Could you check a few things on this model? Use its own coordinates, in mm. Face numbers are marked on the shaded views. A direction names the side the tool comes from. Coordinates: 2 decimals unless noted, no trailing zeros. Loops run counter-clockwise (first coordinate to the right, second up) from the corner with the lowest first, then second, coordinate; pieces in that order, holes last. Notation, with made-up numbers: (62.25, -10.75) - (75.25, -10.75) arc R16 ccw to (75.25, 1.25) - close; hole circle Ø10 at (88, 45). An arc over 180 degrees is marked (long way). Put each result on its own line as item: value. Start each with the question number.
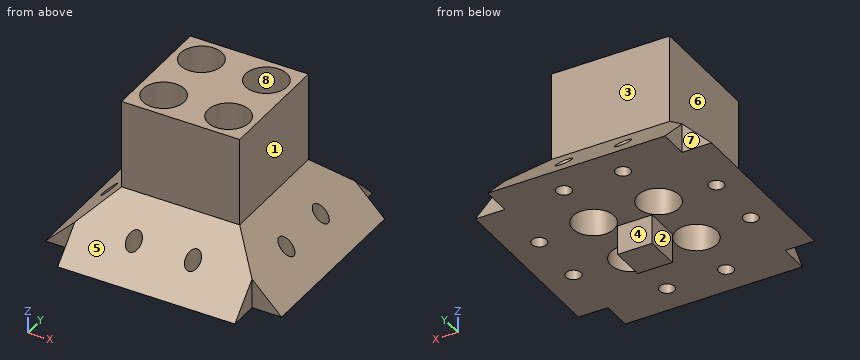
```python
from build123d import *

# Parameters (mm, degrees)
SKETCH_1_W                = 20
SKETCH_1_H                = 20
EXTRUDE_1_DEPTH           = 40
SKETCH_2_W                = 10
SKETCH_2_H                = 15
CUT_EXTRUDE_1_DEPTH       = 7.071067812
PATTERN_CIRCULAR_1_COUNT  = 4
SKETCH_5_R                = 3.5
CUT_EXTRUDE_2_DEPTH       = 25
CUT_EXTRUDE_3_DEPTH       = 5
SKETCH_9_W                = 5.878932188
SKETCH_9_H                = 5.878932188
CUT_EXTRUDE_5_DEPTH       = 5
SKETCH_11_W               = 10
SKETCH_11_H               = 30
EXTRUDE_2_DEPTH           = 10
CUT_EXTRUDE_6_DEPTH       = 30
SKETCH_13_R               = 1.25
CUT_EXTRUDE_7_DEPTH       = 10
PATTERN_CIRCULAR_2_COUNT  = 4
SKETCH_16_W               = 20
SKETCH_16_H               = 10
CUT_EXTRUDE_11_DEPTH      = 40
SKETCH_17_W               = 20
SKETCH_17_H               = 20
SKETCH_17_W_2             = 5.857864376
SKETCH_17_H_2             = 5.857864376
CUT_EXTRUDE_12_DEPTH      = 5
CUT_EXTRUDE_13_DEPTH      = 54.851648071
CUT_EXTRUDE_13_DEPTH_BACK = 10


with BuildPart() as part:
    # 스케치1 → 보스-돌출1 (new body)
    with BuildSketch(Plane.XY):
        Rectangle(SKETCH_1_W, SKETCH_1_H)
    extrude(amount=EXTRUDE_1_DEPTH)

    # 스케치2 → 컷-돌출1 (cut)
    with BuildSketch(Plane(origin=(10, 0, 0), x_dir=(0, 0, -1), z_dir=(1, 0, 0))):
        with Locations((-10, 0)):
            Rectangle(SKETCH_2_W, SKETCH_2_H)
    cut_extrude_1 = extrude(amount=-CUT_EXTRUDE_1_DEPTH, mode=Mode.SUBTRACT)

    # 원형 패턴1: 컷-돌출1 ×4 about axis
    pattern_circular_1_axis = Axis((0, 0, 0), (0, 0, 1))
    for i in range(1, PATTERN_CIRCULAR_1_COUNT):
        add(cut_extrude_1.rotate(pattern_circular_1_axis, i * 360 / PATTERN_CIRCULAR_1_COUNT), mode=Mode.SUBTRACT)

    # 스케치5 → 컷-돌출2 (cut)
    with BuildSketch(Plane.XY.offset(40)):
        with Locations((-5.5, 5.5)):
            Circle(SKETCH_5_R)
        with Locations((5.5, 5.5)):
            Circle(SKETCH_5_R)
        with Locations(Location((-5.5, -5.5, 0), (0, 0, 235.150095421))):
            Circle(SKETCH_5_R)
        with Locations(Location((5.5, -5.5, 0), (0, 0, 304.849904579))):
            Circle(SKETCH_5_R)
    extrude(amount=-CUT_EXTRUDE_2_DEPTH, mode=Mode.SUBTRACT)

    # 스케치6 → 컷-돌출3 (cut)
    with BuildSketch(Plane(origin=(0, 0, 0), x_dir=(-1, 0, 0), z_dir=(0, 0, -1))):
        Polygon((-14.808802863, -2.95), (-14.808802863, 2.95), (-2.95, 2.95), (-2.95, 12.360254216), (2.95, 12.360254216), (2.95, 2.95), (13.852115441, 2.95), (13.852115441, -2.95), (2.95, -2.95), (2.95, -13.975695818), (-2.95, -13.975695818), (-2.95, -2.95), align=None)
    extrude(amount=-CUT_EXTRUDE_3_DEPTH, mode=Mode.SUBTRACT)

    # 스케치9 → 컷-돌출5 (cut)
    with BuildSketch(Plane(origin=(0, 0, 5), x_dir=(-1, 0, 0), z_dir=(0, 0, -1))):
        with Locations((0.010533906, -0.010533906)):
            Rectangle(SKETCH_9_W, SKETCH_9_H)
    extrude(amount=-CUT_EXTRUDE_5_DEPTH, mode=Mode.SUBTRACT)

    # 스케치11 → 보스-돌출2 (add)
    with BuildSketch(Plane(origin=(10, 0, 0), x_dir=(0, 0, -1), z_dir=(1, 0, 0))):
        with Locations((-20, 0)):
            Rectangle(SKETCH_11_W, SKETCH_11_H)
    extrude_2 = extrude(amount=EXTRUDE_2_DEPTH)

    # 스케치12 → 컷-돌출6 (cut)
    with BuildSketch(Plane(origin=(0, 15, 0), x_dir=(1, 0, 0), z_dir=(0, 1, 0))):
        Polygon((20, -15), (10, -25), (20, -25), align=None)
    cut_extrude_6 = extrude(amount=-CUT_EXTRUDE_6_DEPTH, mode=Mode.SUBTRACT)

    # 스케치13 → 컷-돌출7 (cut)
    with BuildSketch(Plane(origin=(0, 0, 15), x_dir=(-1, 0, 0), z_dir=(0, 0, -1))):
        with Locations(Location((-15, -5, 0), (0, 0, 90))):
            Circle(SKETCH_13_R)
        with Locations(Location((-15, 5, 0), (0, 0, 90))):
            Circle(SKETCH_13_R)
    cut_extrude_7 = extrude(amount=-CUT_EXTRUDE_7_DEPTH, mode=Mode.SUBTRACT)

    # 원형 패턴2: 보스-돌출2, 컷-돌출6, 컷-돌출7 ×4 about axis
    pattern_circular_2_axis = Axis((0, 0, 0), (0, 0, 1))
    add([extrude_2.rotate(pattern_circular_2_axis, i * 360 / PATTERN_CIRCULAR_2_COUNT) for i in range(1, PATTERN_CIRCULAR_2_COUNT)])
    add([cut_extrude_6.rotate(pattern_circular_2_axis, i * 360 / PATTERN_CIRCULAR_2_COUNT) for i in range(1, PATTERN_CIRCULAR_2_COUNT)], mode=Mode.SUBTRACT)
    add([cut_extrude_7.rotate(pattern_circular_2_axis, i * 360 / PATTERN_CIRCULAR_2_COUNT) for i in range(1, PATTERN_CIRCULAR_2_COUNT)], mode=Mode.SUBTRACT)

    # 스케치16 → 컷-돌출11 (cut)
    with BuildSketch(Plane.XZ.offset(10)):
        with Locations((0, 5)):
            Rectangle(SKETCH_16_W, SKETCH_16_H)
    extrude(amount=-CUT_EXTRUDE_11_DEPTH, mode=Mode.SUBTRACT)

    # 스케치17 → 컷-돌출12 (cut)
    with BuildSketch(Plane(origin=(0, 0, 10), x_dir=(-1, 0, 0), z_dir=(0, 0, -1))):
        Rectangle(SKETCH_17_W, SKETCH_17_H)
        Rectangle(SKETCH_17_W_2, SKETCH_17_H_2, mode=Mode.SUBTRACT)
    extrude(amount=-CUT_EXTRUDE_12_DEPTH, mode=Mode.SUBTRACT)

    # 스케치18 → 컷-돌출13 (cut, two sides: drawn at the far end of the back side and taken through both)
    with BuildSketch(Plane.XZ.offset(-10).offset(-CUT_EXTRUDE_13_DEPTH_BACK)):
        Polygon((10, 25), (15, 25), (15, 20), align=None)
    extrude(amount=CUT_EXTRUDE_13_DEPTH + CUT_EXTRUDE_13_DEPTH_BACK, mode=Mode.SUBTRACT)


solid = part.part
```
(1) For pin 1 Ø3 at (x, y) = (5, 15) entering from -Z; pin 2 Ø5.5 at (y, z) = (16.5, 18.5) entering from -X; pin 3 Ø12 at (y, z) = (9, 35.5) entering from -X, each with a flat end and sliding along its axis, tell me the tip position at first contact or that it passes through.
(2) Which directions (+Z, -Z, +X, -X, +Y, -Y) give clear straight access to the entire face, cutting with the end or side of a thin tool? Please do the marked faces 1, 2, 3 and 4.
(3) I want a section at C-C on x = -5.5. List the corners of the cut face in (y, z) for me.
(4) I want a section at A-A on y = -5. List the corners of the cut face in (x, z) for me.
(5) I want a section at D-D on x = -0.5. List the corners of the cut face in (y, z) for me.
(6) I need wall thicknesses on L1, parallel to Y at x = -5, z = 19; L2, parallel to X at y = 8.5, z = 15.25; L3, parallel to Y at x = 8, z = 34.25. Which ranges of each line are inside material? Lowest first, please. Write a range as [from, to].
(7) If we mould it in two halves opening along Y, with no side actions, what happens to the marked faces 5, 6, 7 and 8? For each: pulls with the +Y half, pulls with the -Y half, needs draft (parallel to the pull), parting line crosses it, or undercut.
(8) I want a section at B-B on z = 37.75. List the corners of the cut face in (x, y) for me, and give its area (3 significant figures).
Answer sheet:
1. pin 1: stops at z = 15
1. pin 2: stops at x = -18.8
1. pin 3: stops at x = -10
2. face 1: +Z, +X, +Y, -Y
2. face 2: -Z, -X, +Y, -Y
2. face 3: +Z, +X, -X, +Y
2. face 4: -Z, +X, -X, +Y
3. outline: (-20, 15) - (-16.15, 15) - (-16.15, 18.85) - close; (-13.85, 15) - (-9, 15) - (-9, 40) - (-10, 40) - (-10, 25) - (-13.85, 21.15) - close; (-2, 15) - (2, 15) - (2, 40) - (-2, 40) - close; (9, 15) - (13.85, 15) - (13.85, 21.15) - (10, 25) - (10, 40) - (9, 40) - close; (16.15, 15) - (20, 15) - (16.15, 18.85) - close
4. outline: (-20, 15) - (-16.25, 15) - (-16.25, 18.75) - close; (-13.75, 15) - (-8.96, 15) - (-8.96, 40) - (-10, 40) - (-10, 25) - (-13.75, 21.25) - close; (-2.04, 15) - (2.04, 15) - (2.04, 40) - (-2.04, 40) - close; (8.96, 15) - (13.75, 15) - (13.75, 21.25) - (10, 25) - (10, 40) - (8.96, 40) - close; (16.25, 15) - (20, 15) - (16.25, 18.75) - close
5. outline: (-20, 15) - (-2.93, 15) - (-2.93, 10) - (2.93, 10) - (2.93, 15) - (20, 15) - (10, 25) - (10, 40) - (-10, 40) - (-10, 25) - close
6. L1: y = [-13.75, -8.96], [-2.04, 2.04], [8.96, 13.75]
6. L2: x = [-19.75, -7.3], [-3.7, 3.7], [7.3, 19.75]
6. L3: y = [-10, -7.95], [-3.05, 3.05], [7.95, 10]
7. face 5: pulls with the -Y half
7. face 6: needs draft
7. face 7: pulls with the +Y half
7. face 8: undercut
8. outline: (-10, -10) - (10, -10) - (10, 10) - (-10, 10) - close; hole circle Ø7 at (-5.5, -5.5); hole circle Ø7 at (-5.5, 5.5); hole circle Ø7 at (5.5, -5.5); hole circle Ø7 at (5.5, 5.5)
8. area: 246 mm^2
